Here's the drawing with two shaded views (mm, measured from the low corner). I have some questions. A direction names the side the tool comes from. Coordinates: 2 decimals unless noted, no trailing zeros. Order: outer loops, then holes, each group sorted by start corner. A loop starts at its lowest first (then second) coordinate and runs counter-clockwise, first axis right, second up. Notation, with made-up numbers: (26, 12.25) - (84, 12.25) arc R17 cw to (84, 25.25) - close; hole circle Ø1 at (43.25, 83.5). An arc over 180 degrees is marked (long way). One line per item, written item: value. Start each with the question number.
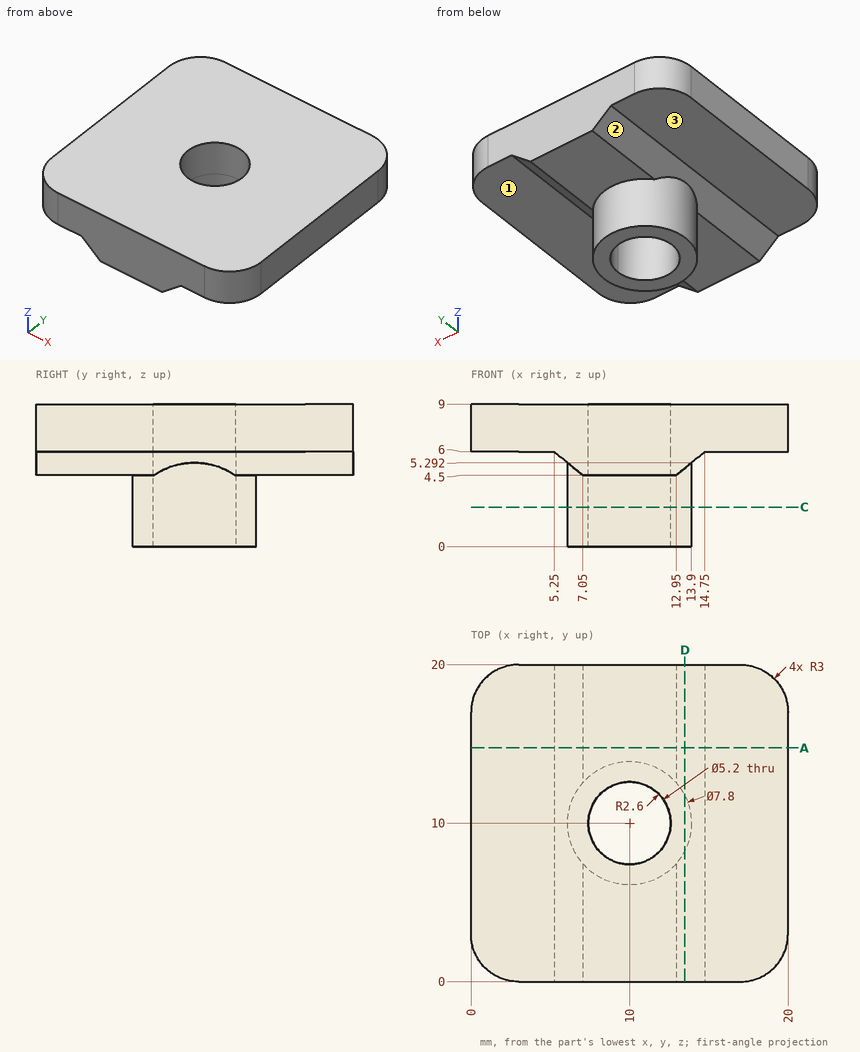
Q1. I'm going to push flat-ended pins straight in: pin 1 (4.5 mm diameter, centred on x = 10, y = 10, fed in from -Z); pin 2 (4 mm diameter, centred on x = 17, y = 6, fed in from -Z); pin 3 (6 mm diameter, centred on x = 15.5, y = 3, fed in from -Z); pin 4 (1.5 mm diameter, centred on y = 16, z = 5, fed in from +X). Where does each tip first touch, or does it pass through?
Q2. If I drill on L1, parallel to Y at x = 10, z = 1.85; L2, parallel to Y at x = 10, z = 7.35, over which ranges is the centre line in solid material (lowest first)?
Q3. Which directions (+Z, -Z, +X, -X, +Y, -Y) give clear straight access to the entire face, cutting with the end or side of a thin tool? Please do the marked faces 1, 2 and 3.
Q4. I want a section at A-A on y = 14.75. Please give me the cut outline in (x, z).
Q5. I want a section at D-D on x = 13.5. Please give me the cut outline in (y, z), then the cut area to 3 significant figures.
Q6. I want a section at C-C on z = 2.5. Please give me the cut outline in (x, y).
Values follow:
1. pin 1: passes through
1. pin 2: stops at z = 6
1. pin 3: stops at z = 4.5
1. pin 4: stops at x = 14.45
2. L1: y = 6.1 to 7.4, 12.6 to 13.9
2. L2: y = 0 to 7.4, 12.6 to 20
3. face 1: -Z, +X, +Y, -Y
3. face 2: -Z, -X
3. face 3: -Z, -X, +Y, -Y
4. outline: (0, 6) - (5.25, 6) - (7.05, 4.5) - (12.95, 4.5) - (14.75, 6) - (20, 6) - (20, 9) - (0, 9) - close
5. outline: (0, 4.96) - (8.28, 4.96) - (8.28, 0) - (11.72, 0) - (11.72, 4.96) - (20, 4.96) - (20, 9) - (0, 9) - close
5. area: 97.9 mm^2
6. outline: circle Ø7.8 at (10, 10); hole circle Ø5.2 at (10, 10)
